Check sheet for the modelled part. Datum: model origin and axes. Units: mm. Face numbers are marked on the shaded views. A direction names the side the tool comes from. Round coordinates to 2 decimals unless told otherwise and drop trailing zeros. Loops run counter-clockwise (first coordinate to the right, second up) from the corner with the lowest first, then second, coordinate; pieces in that order, holes last. Notation, with made-up numbers: (13.5, 73.25) - (65.5, 73.25) arc R27 ccw to (65.5, 93.25) - close; hole circle Ø5 at (65.5, 50). An arc over 180 degrees is marked (long way). Answer in a Markdown table with one row per item. Add a question column.
(1) Cross-section at D-D on y = 55. Enter the section's corners in (x, z).
(2) Cross-section at B-B on x = 0. Enter the section's corners in (y, z), then the cut area to 3 significant figures.
(3) Gauge pin test, flat end, axial feed: pin 1 (2 mm diameter, centred on x = 1, y = -15.5, fed in from +Z). Record the tip position at first contact, or that the pin passes through.
(4) Cross-section at A-A on z = 4. Enter the section's corners in (x, y).
(5) Mould release check, pull along Y, two halves, no side actions. Record for the marked faces 4, 5 and 6: +Y half, -Y half, draft (parallel to the pull), parting line (faces both ways), or undercut.
(6) Cross-section at C-C on y = -35.5. Enter the section's corners in (x, z), then the cut area to 3 significant figures.
(7) Thickness scan on line 1 along Y through (x, z) = (1.25, 7); line 2 along Y through (x, z) = (4, 4.5); line 3 along Y through (x, z) = (-6, 0.75). Record the ranges inside material, lowest first.
(8) Access from +Z, -Z, +X, -X, +Y, -Y to the whole of each face (thin tool, end or side, straight path). Record for the marked faces 1, 2 and 3.
from build123d import *

# Parameters (mm, degrees)
F0_W     = 12.5
F0_H     = 7
F1_DEPTH = 8
F0_W_2   = 6.5
F0_H_2   = 15
F0_H_3   = 4
F2_DEPTH = 2.5


# Not quite as in the source:
# - a feature names something its author has since deleted; it is built from what else it names


with BuildPart() as f1:
    # F0 (on Top) → F1 (new body)
    with BuildSketch(Plane.XY):
        Polygon((-6.0006843501, 44.5469320043), (-5.9425927878, 44.5469320043), (-5.9425927878, 71.5469320043), (-5.9425927878, 78.5469320043), (-11, 78.5469320043), (-11, 44.5469320043), align=None)
        Polygon((11, -44.5469320043), (11, 44.5469320043), (1.4993156499, 44.5469320043), (-5.9425927878, 44.5469320043), (-6.0006843501, 44.5469320043), (-11, 44.5469320043), (-11, -44.5469320043), align=None)
        Polygon((-3.25, -4.2208939195), (3.25, -4.2208939195), (3.25, -19.2208939195), (8.25, -19.2208939195), (8.25, -23.2208939195), (3.25, -23.2208939195), (3.25, -38.2208939195), (-3.25, -38.2208939195), (-3.25, -23.2208939195), (-8.25, -23.2208939195), (-8.25, -19.2208939195), (-3.25, -19.2208939195), align=None, mode=Mode.SUBTRACT)
        with Locations((0.3074072122, 75.0469320043)):
            Rectangle(F0_W, F0_H)
    extrude(amount=F1_DEPTH)

    # F0 (on Top) → F2 (join)
    with BuildSketch(Plane.XY):
        with Locations((0, -11.7208939195)):
            Rectangle(F0_W_2, F0_H_2)
        with Locations((0, -21.2208939195)):
            Rectangle(F0_W_2, F0_H_3)
        with Locations((0, -30.7208939195)):
            Rectangle(F0_W_2, F0_H_2)
    extrude(amount=F2_DEPTH)


solid = f1.part
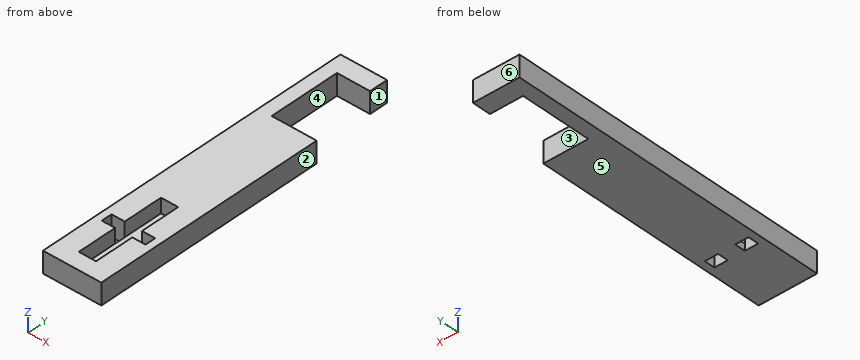
Answers:
| question | item | result |
|---|---|---|
| 1 | outline | (-11, 0) - (-5.94, 0) - (-5.94, 8) - (-11, 8) - close |
| 2 | outline | (-44.55, 0) - (44.55, 0) - (44.55, 8) - (-4.22, 8) - (-4.22, 2.5) - (-38.22, 2.5) - (-38.22, 8) - (-44.55, 8) - close; (71.55, 0) - (78.55, 0) - (78.55, 8) - (71.55, 8) - close |
| 2 | area | 582 mm^2 |
| 3 | pin 1 | stops at z = 2.5 |
| 4 | outline | (-11, -44.55) - (11, -44.55) - (11, 44.55) - (-5.94, 44.55) - (-5.94, 71.55) - (6.56, 71.55) - (6.56, 78.55) - (-11, 78.55) - close; hole (-8.25, -23.22) - (-3.25, -23.22) - (-3.25, -38.22) - (3.25, -38.22) - (3.25, -23.22) - (8.25, -23.22) - (8.25, -19.22) - (3.25, -19.22) - (3.25, -4.22) - (-3.25, -4.22) - (-3.25, -19.22) - (-8.25, -19.22) - close |
| 5 | face 4 | undercut |
| 5 | face 5 | draft |
| 5 | face 6 | +Y half |
| 6 | outline | (-11, 0) - (11, 0) - (11, 8) - (3.25, 8) - (3.25, 2.5) - (-3.25, 2.5) - (-3.25, 8) - (-11, 8) - close |
| 6 | area | 140 mm^2 |
| 7 | line 1 | y = -44.55 to -38.22, -4.22 to 44.55, 71.55 to 78.55 |
| 7 | line 2 | y = -44.55 to -23.22, -19.22 to 44.55, 71.55 to 78.55 |
| 7 | line 3 | y = -44.55 to -23.22, -19.22 to 78.55 |
| 8 | face 1 | +Z, -Z, +X, +Y |
| 8 | face 2 | +Z, -Z, +X, +Y, -Y |
| 8 | face 3 | +Z, -Z, +X |
